Input: part model. Units: mm. Frame: model coordinates. Face numbers are marked on the shaded views. A direction names the side the tool comes from. Round coordinates to 2 decimals unless told otherwise and drop trailing zeros. Write each loop counter-clockwise with the first axis right and the second up, starting at its lowest first coordinate (ties: lowest second). Pieces come first, ordered by that corner, then holes. Notation, with made-up numbers: M -3.5,70.5 L 33.5,70.5 A31 ccw 33.5,107.5 Z; hole C 58,15 d5. An arc over 180 degrees is marked long. Use one line per item in the form item = value. Start each with the question number.
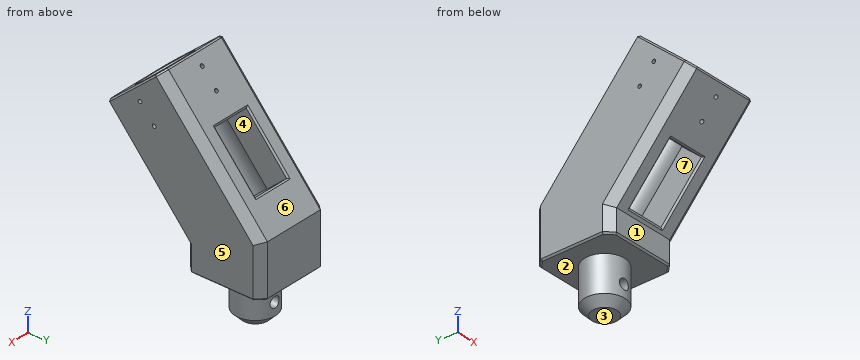
```python
from build123d import *

# Parameters (mm, degrees)
F0_W      = 50
F0_H      = 50
F1_DEPTH  = 15
F2_R      = 12.9
F3_DEPTH  = 28
F4_R      = 3.4
F5_DEPTH  = 21
F7_DEPTH  = 50
F8_R      = 14
F9_DEPTH  = 77
F10_R     = 16.1
F11_DEPTH = 30
F12_W     = 24
F12_H     = 40
F13_DEPTH = 117.8222610619
F14_R     = 1.2
F15_DEPTH = 117.8222610619
F16_R     = 1.2
F17_DEPTH = 50.001
F18_SIZE  = 5
F19_SIZE  = 1


with BuildPart() as f1:
    # F0 (on Top) → F1 (new body)
    with BuildSketch(Plane.XY):
        Rectangle(F0_W, F0_H)
    extrude(amount=F1_DEPTH)

    # F2 (on face) → F3 (join)
    with BuildSketch(Plane(origin=(0, 0, 0), x_dir=(1, 0, 0), z_dir=(0, 0, -1))):
        Circle(F2_R)
    extrude(amount=F3_DEPTH)

    # F4 (on Front) → F5 (cut, symmetric)
    with BuildSketch(Plane.XZ):
        with Locations((0, -15)):
            Circle(F4_R)
    extrude(amount=F5_DEPTH, both=True, mode=Mode.SUBTRACT)

    # F6 (on face) → F7 (join)
    with BuildSketch(Plane.YZ.offset(25)):
        Polygon((-77.4847223192, 75.3767664178), (-25, 15), (25, 15), (25, 33.6942339742), (-39.7492433081, 108.1797178673), align=None)
    extrude(amount=-F7_DEPTH)

    # F8 (on face) → F9 (cut)
    with BuildSketch(Plane(origin=(0, -70.6720690728, 81.2989155343), x_dir=(1, 0, 0), z_dir=(0, -0.656059029, 0.7547095802))):
        with Locations((0, 15.9731459293)):
            Circle(F8_R)
    extrude(amount=-F9_DEPTH, mode=Mode.SUBTRACT)

    # F10 (on face) → F11 (cut)
    with BuildSketch(Plane(origin=(0, -70.6720690728, 81.2989155343), x_dir=(1, 0, 0), z_dir=(0, -0.656059029, 0.7547095802))):
        with Locations((0, 15.9731459293)):
            Circle(F10_R)
    extrude(amount=-F11_DEPTH, mode=Mode.SUBTRACT)

    # F12 (on face) → F13 (cut, through all)
    with BuildSketch(Plane(origin=(0, 30.9228257647, 26.8808023331), x_dir=(-1, 0, 0), z_dir=(0, 0.7547095802, 0.656059029))):
        with Locations((0, 50.7221194281)):
            Rectangle(F12_W, F12_H)
    extrude(amount=-F13_DEPTH, mode=Mode.SUBTRACT)

    # F14 (on face) → F15 (cut, through all)
    with BuildSketch(Plane(origin=(0, 30.9228257647, 26.8808023331), x_dir=(-1, 0, 0), z_dir=(0, 0.7547095802, 0.656059029))):
        with Locations((0, 99.7221194281)):
            Circle(F14_R)
        with Locations((0, 85.7221194281)):
            Circle(F14_R)
    extrude(amount=-F15_DEPTH, mode=Mode.SUBTRACT)

    # F16 (on face) → F17 (cut, through all)
    with BuildSketch(Plane.YZ.offset(25)):
        with Locations((-53.3685105817, 85.7405655008)):
            Circle(F16_R)
        with Locations((-44.1836841759, 75.1746313777)):
            Circle(F16_R)
    extrude(amount=-F17_DEPTH, mode=Mode.SUBTRACT)

    # F18
    f18_edges = [f1.edges().sort_by_distance(p)[0] for p in [
        (-12.9, 0, -28),
        (25, -51.242361, 45.188383),
        (25, -25, 7.5),
        (25, 25, 16.847117),
        (25, -7.374622, 70.936976),
        (-25, 25, 16.847117),
        (-25, -7.374622, 70.936976),
        (-25, -25, 7.5),
        (-25, -51.242361, 45.188383),
    ]]
    chamfer(f18_edges, length=F18_SIZE)

    # F19
    f19_edges = [f1.edges().sort_by_distance(p)[0] for p in [
        (-16.1, -58.616983, 91.778242),
        (12, -40.089358, 32.35832),
        (0, -53.210538, 47.452512),
        (-12, -40.089358, 32.35832),
        (0, -26.968177, 17.264129),
        (0, 10.767302, 50.06708),
        (-12, -2.353879, 65.161272),
        (12, -2.353879, 65.161272),
        (0, -15.475059, 80.255463),
        (-25, 0, 0),
        (-22.5, -22.5, 0),
        (0, -25, 0),
        (22.5, -22.5, 0),
        (25, 0, 0),
        (22.5, 22.5, 0),
        (0, 25, 0),
        (-22.5, 22.5, 0),
        (0, -77.484722, 75.376766),
        (-22.5, -75.597948, 77.016914),
        (-25, -58.616983, 91.778242),
        (25, -58.616983, 91.778242),
        (22.5, -75.597948, 77.016914),
        (22.5, -41.636017, 106.53957),
        (0, -39.749243, 108.179718),
        (-22.5, -41.636017, 106.53957),
    ]]
    chamfer(f19_edges, length=F19_SIZE)


solid = f1.part
```
Item 1: Cut plane B-B (z = 25.5). Output: boundary loops of the cut face in (x, y).
Item 2: Ray query, line 1 (X direction, y = -34.5, z = 44.5); line 2 (Z direction, x = 0, y = 6.5); line 3 (Z direction, x = -2, y = 12). Return the intervals inside material, ascending. Write a range as from..to.
Item 3: First-contact query: pin 1 (3 mm diameter, centred on x = -12, y = -15.5, fed in from +Z); pin 2 (10 mm diameter, centred on x = -13.5, y = -24.5, fed in from -Z); pin 3 (6 mm diameter, centred on x = 4.5, y = -45, fed in from -Z). Flat tips, straight axial feed; report the tip coordinate or a pass-through.
Item 4: Reachability of the marked faces 1, 2 and 3 from +Z, -Z, +X, -X, +Y, -Y: full face, straight path, thin tool, end or side. Return the list, or none.
Item 5: Cut plane C-C (z = -15). Output: boundary loops of the cut face in (x, y), plus the area to 3 significant figures.
Item 6: Draft query along Z for the marked faces 4, 5, 6 and 7. Return one class per face: +Z half, -Z half, draft (parallel to the pull), parting line (faces both ways), or undercut.
Item 7: Cut plane A-A (y = 0). Output: boundary loops of the cut face in (x, z), plus the area to 3 significant figures.
Final values:
q1.outline = M -25,-27.5 L -20,-34.13 L -13,-34.13 L -12,-32.8 L -12,-17.49 L 12,-17.49 L 12,-32.8 L 13,-34.13 L 20,-34.13 L 25,-27.5 L 25,20 L 20,25 L -20,25 L -25,20 Z
q2.line_1 = -25..-12, 12..25
q2.line_2 = -28..-18.4, -11.6..46.36
q2.line_3 = -23.73..-17.75, -12.25..48.65
q3.pin_1 = 82.01
q3.pin_2 = 0
q3.pin_3 = 51.98
q4.face_1 = -Z, +X, -X, -Y
q4.face_2 = -Z
q4.face_3 = -Z, +X, -X, +Y, -Y
q5.outline = M -3.4,-12.44 L -3.4,12.44 A12.9 ccw Z; M 3.4,-12.44 A12.9 ccw 3.4,12.44 Z
q5.area = 349 mm^2
q6.face_4 = undercut
q6.face_5 = draft
q6.face_6 = +Z half
q6.face_7 = undercut
q7.outline = M -25,1 L -24,0 L -12.9,0 L -12.9,-23 L -7.9,-28 L 7.9,-28 L 12.9,-23 L 12.9,0 L 24,0 L 25,1 L 25,54.83 L 20,62.45 L 13,62.45 L 12,60.93 L 12,40.71 L -12,40.71 L -12,60.93 L -13,62.45 L -20,62.45 L -25,54.83 Z; hole C 0,-15 d6.8
q7.area = 3,220 mm^2
